from build123d import *

# Parameters (mm, degrees)
SKETCH1_W               = 127
SKETCH1_H               = 6.35
BOSS_EXTRUDE1_DEPTH     = 127
CUT_EXTRUDE1_DEPTH      = 1
CUT_EXTRUDE1_DEPTH_BACK = 7.35


with BuildPart() as part:
    # Sketch1 → Boss-Extrude1 (new body)
    with BuildSketch(Plane.XY):
        Rectangle(SKETCH1_W, SKETCH1_H)
    extrude(amount=BOSS_EXTRUDE1_DEPTH)

    # Sketch2 → Cut-Extrude1 (cut, two sides)
    with BuildSketch(Plane.XZ.offset(3.175)) as cut_extrude1_sk:
        Polygon((63.5, 63.5), (46.485226281, 127), (63.5, 127), align=None)
    extrude(amount=CUT_EXTRUDE1_DEPTH, mode=Mode.SUBTRACT)
    extrude(cut_extrude1_sk.sketch, amount=-CUT_EXTRUDE1_DEPTH_BACK, mode=Mode.SUBTRACT)


solid = part.part
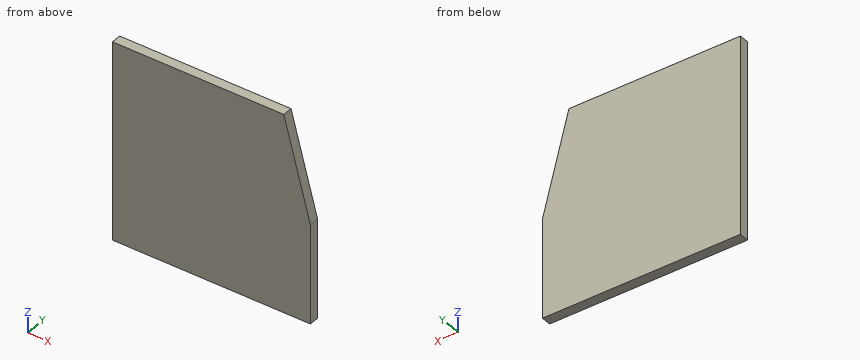
CAD build for the part. Positions are in the model's coordinates, mm. Round coordinates to 2 decimals unless told otherwise and drop trailing zeros. Loops run counter-clockwise (first coordinate to the right, second up) from the corner with the lowest first, then second, coordinate; pieces in that order, holes last.
(1) Cut at B-B (x = 51). Give the cut face in (y, z) (3 decimals), plus the area to 3 significant figures.
(2) Wall check: line 1 along X through (y, z) = (-1.25, 96.5); line 2 along X through (y, z) = (0, 70). Give the ranges that are in metal, low to high.
(3) Cut at A-A (y = -0.75). Give the cut face in (x, z), plus the area to 3 significant figures.
(4) Cut at C-C (z = 97). Give the cut face in (x, y) (3 decimals).
Findings below:
1. outline: (-3.175, 0) - (3.175, 0) - (3.175, 110.151) - (-3.175, 110.151) - close
1. area: 699 mm2
2. line 1: x = -63.5 to 54.66
2. line 2: x = -63.5 to 61.76
3. outline: (-63.5, 0) - (63.5, 0) - (63.5, 63.5) - (46.49, 127) - (-63.5, 127) - close
3. area: 15,600 mm2
4. outline: (-63.5, -3.175) - (54.524, -3.175) - (54.524, 3.175) - (-63.5, 3.175) - close
